Print and shaded views of the part. All mm, measured from the part's lowest x, y and z. A direction names the side the tool comes from. Give positions to 0.01 mm unless a question says otherwise; leave off trailing zeros. Loops run counter-clockwise (first coordinate to the right, second up) from the corner with the lowest first, then second, coordinate; pieces in that order, holes last. Notation, with made-up numbers: (76.25, 38.25) - (99.25, 38.25) arc R18 cw to (99.25, 71.25) - close; hole circle Ø6 at (45.5, 82). An arc over 180 degrees is marked (long way). Return JSON: item names as keys, results as strings.
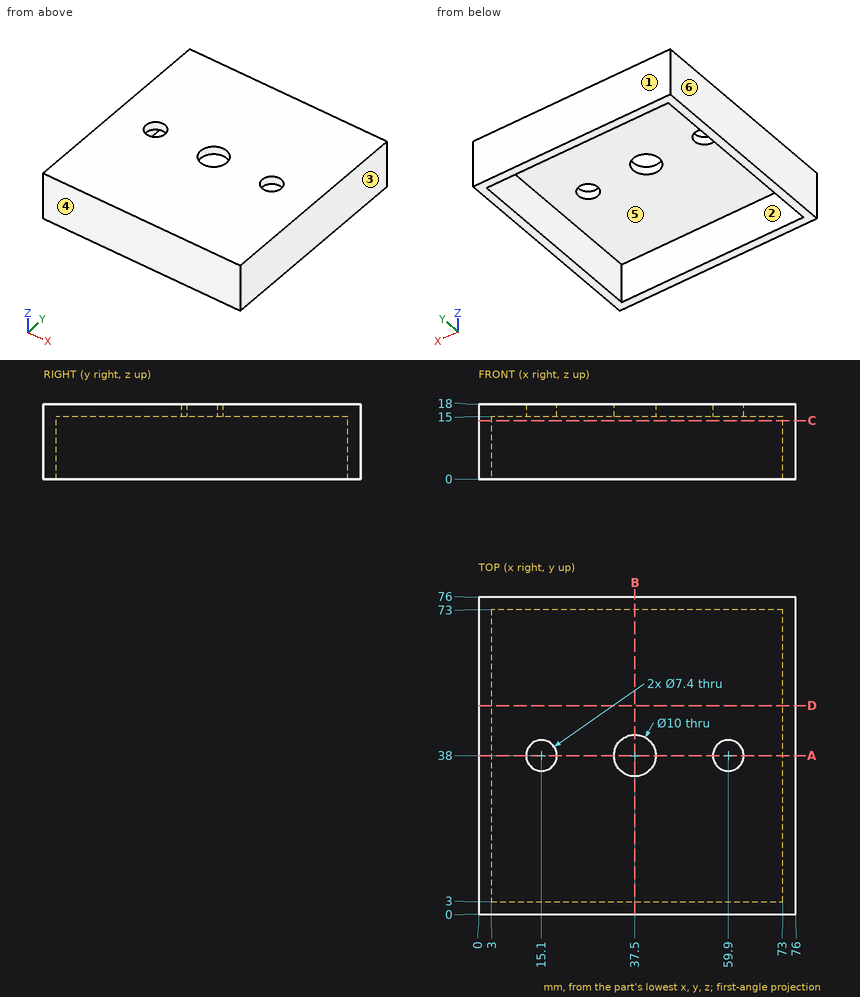
1. Which spindle directions (+Z, -Z, +X, -X, +Y, -Y) get a long thin tool onto all of the face, cutting with end or side? Do the marked faces 1 and 2. Say none if no direction does.
Values follow:
{"face 1": "+Z, -Z, +X, -X, +Y", "face 2": "-Z"}
2. Cut at A-A, the plane y = 38. Write the cut outline in (x, z).
Values follow:
{"outline": "(0, 0) - (3, 0) - (3, 15) - (11.4, 15) - (11.4, 18) - (0, 18) - close; (18.8, 15) - (32.5, 15) - (32.5, 18) - (18.8, 18) - close; (42.5, 15) - (56.2, 15) - (56.2, 18) - (42.5, 18) - close; (63.6, 15) - (73, 15) - (73, 0) - (76, 0) - (76, 18) - (63.6, 18) - close"}
3. Drop flat-ended pins along their axis: P1, Ø6, axis at x = 37.5, y = 38, coming from the +Z side; P2, Ø6, axis at x = 23.5, y = 36, coming from the -Z side. Give the stop position or say it passes through.
Values follow:
{"P1": "passes through", "P2": "stops at z = 15"}
4. Drill centre lines: probe 1 along Y at (x, z) = (62, 8.25); probe 2 along Y at (x, z) = (15.1, 16.3). Where is each one in solid material? Low to high.
Values follow:
{"probe 1": "y = 0 to 3, 73 to 76", "probe 2": "y = 0 to 34.3, 41.7 to 76"}
5. Cut at D-D, the plane y = 50. Write the cut outline in (x, z), plus the area to 3 significant figures.
Values follow:
{"outline": "(0, 0) - (3, 0) - (3, 15) - (73, 15) - (73, 0) - (76, 0) - (76, 18) - (0, 18) - close", "area": "318 mm²"}
6. Cut at C-C, the plane z = 14. Write the cut outline in (x, y).
Values follow:
{"outline": "(0, 0) - (76, 0) - (76, 76) - (0, 76) - close; hole (3, 3) - (73, 3) - (73, 73) - (3, 73) - close"}
7. Pull direction X, two halves, no side cores. Call the marked faces 3, 4, 5 and 6: +X half, -X half, draft (parallel to the pull), parting line (faces both ways), or undercut.
Values follow:
{"face 3": "+X half", "face 4": "draft", "face 5": "undercut", "face 6": "-X half"}
8. Cut at B-B, the plane x = 37.5. Write the cut outline in (y, z).
Values follow:
{"outline": "(0, 0) - (3, 0) - (3, 15) - (33, 15) - (33, 18) - (0, 18) - close; (43, 15) - (73, 15) - (73, 0) - (76, 0) - (76, 18) - (43, 18) - close"}
